from build123d import *

# Parameters (mm, degrees)
SKETCH_1_R               = 10
SKETCH_1_R_2             = 8.5
EXTRUDE_325_DEPTH        = 28
SKETCH_2_R               = 2
CUT_EXTRUDE_1_DEPTH      = 32.368774283
PATTERN_CIRCULAR_1_COUNT = 2
PATTERN_CIRCULAR_1_ANGLE = 120


with BuildPart() as part:
    # Эскиз1 → Extrude 325 (new body)
    with BuildSketch(Plane(origin=(0, 0, 0), x_dir=(1, 0, 0), z_dir=(0, 1, 0))):
        with Locations(Location((0, 0, 0), (0, 0, 270))):
            Circle(SKETCH_1_R)
        with Locations(Location((0, 0, 0), (0, 0, 270))):
            Circle(SKETCH_1_R_2, mode=Mode.SUBTRACT)
    extrude(amount=EXTRUDE_325_DEPTH)

    # Эскиз2 → отверстие чтоб прикрутиться 1 (cut, through all)
    with BuildSketch(Plane.XY):
        with Locations(Location((0, 4.5, 0), (0, 0, 269.999999945))):
            Circle(SKETCH_2_R)
    cut_extrude_1 = extrude(amount=CUT_EXTRUDE_1_DEPTH, mode=Mode.SUBTRACT)

    # Круговой массив1: отверстие чтоб прикрутиться 1 ×2 about axis
    pattern_circular_1_axis = Axis((0, 28, 0), (0, -1, 0))
    for i in range(1, PATTERN_CIRCULAR_1_COUNT):
        add(cut_extrude_1.rotate(pattern_circular_1_axis, i * PATTERN_CIRCULAR_1_ANGLE / (PATTERN_CIRCULAR_1_COUNT - 1)), mode=Mode.SUBTRACT)


solid = part.part
The listing builds one solid part. Answer for the finished solid, in the listing's coordinates (mm). Coordinates: 2 decimals unless noted, no trailing zeros. Write each loop counter-clockwise with the first axis right and the second up, starting at its lowest first coordinate (ties: lowest second). Pieces come first, ordered by that corner, then holes. Notation, with made-up numbers: (66.25, 5.5) -> (86.25, 5.5) arc R17 cw to (86.25, 11.5) -> close; hole circle Ø3 at (27, 79). An arc over 180 degrees is marked (long way). One line per question, with ' | ' between items.
1. Section C-C (x = 5.5) is taken. Determine the outline of the cut face in (y, z), and give its area (3 significant figures).
Verdict:
outline: (0, -8.35) -> (28, -8.35) -> (28, -6.48) -> (0, -6.48) -> close; (0, 6.48) -> (28, 6.48) -> (28, 8.35) -> (0, 8.35) -> close | area: 105 mm^2
2. Section D-D (y = 14.25) is taken. Determine the outline of the cut face in (x, z), and give its area (3 significant figures).
Verdict:
outline: circle Ø20 at (0, 0); hole circle Ø17 at (0, 0) | area: 87.2 mm^2
3. For a pull along X with two mould halves and no side action, classify faces 1 (the cylindrical face through (-9.76, 13.8, -2.17)), 2 (the flat face through (-7.4, 0, -4.5)), 3 (the cylindrical face through (0.601, 2.592, 9.119)), 4 (the cylindrical face through (8.428, 13.804, -1.107)) as released by +X, released by -X, zero draft, split by the parting line, or undercut.
Verdict:
face 1: split by the parting line | face 2: zero draft | face 3: undercut | face 4: undercut
4. Section B-B (x = 0) is taken. Determine the outline of the cut face in (y, z), and give its area (3 significant figures).
Verdict:
outline: (0, -10) -> (28, -10) -> (28, -8.5) -> (0, -8.5) -> close; (0, 8.5) -> (2.5, 8.5) -> (2.5, 10) -> (0, 10) -> close; (6.5, 8.5) -> (28, 8.5) -> (28, 10) -> (6.5, 10) -> close | area: 78.0 mm^2
5. Given pin 1 Ø1.5 at (y, z) = (13, -2) entering from +X; pin 2 Ø5 at (y, z) = (5.5, 5.5) entering from -X, each flat-ended and moving along its own axis, determine where each tip first touches the part or whether it passes through.
Verdict:
pin 1: stops at x = 9.92 | pin 2: stops at x = -9.54
6. Straight lines are drawn through the part: line 1 (X direction, y = 22.25, z = 0); line 2 (Y direction, x = 0, z = 8.75); line 3 (X direction, y = 12, z = -6.5). For each, find the intervals that lie inside material, in ascending order.
Verdict:
line 1: x = -10 to -8.5, 8.5 to 10 | line 2: y = 0 to 2.5, 6.5 to 28 | line 3: x = -7.6 to -5.48, 5.48 to 7.6
7. Section A-A (z = 0) is taken. Determine the outline of the cut face in (x, y), and give its area (3 significant figures).
Verdict:
outline: (-10, 0) -> (-8.5, 0) -> (-8.5, 28) -> (-10, 28) -> close; (8.5, 0) -> (10, 0) -> (10, 28) -> (8.5, 28) -> close | area: 84.0 mm^2
